CAD build for the part. Positions are in the model's coordinates, mm. Round coordinates to 2 decimals unless told otherwise and drop trailing zeros. Loops run counter-clockwise (first coordinate to the right, second up) from the corner with the lowest first, then second, coordinate; pieces in that order, holes last.
Autodesk Fusion 360 part; units mm, degrees
sketch "Sketch1" plane through (0, 0, 0) normal (0, 0, 1) x (1, 0, 0)
  line L0 (0, 0) -> (10, 0)
  line L1 (10, 0) -> (10, 10)
  line L2 (10, 10) -> (0, 10)
  line L3 (0, 10) -> (0, 0)
extrude "Extrude1" add sketch "Sketch1" along normal blind 10
fillet "Fillet1" radius 10 1 edges at (0, 5, 10)
Item 1: Cut at B-B, the plane x = 5.75. Give the cut face in (y, z).
Answers follow:
outline: (0, 0) - (10, 0) - (10, 9.05) - (0, 9.05) - close
Item 2: Probe line 1 (X direction, y = 6.5, z = 5.5); line 2 (Z direction, x = 9, y = 4.75); line 3 (Z direction, x = 2.75, y = 2). List the from-to ranges inside material, lowest first.
Answers follow:
line 1: x = 1.65 to 10
line 2: z = 0 to 9.95
line 3: z = 0 to 6.89
Item 3: Flat gauge pins, fed straight in: P1, Ø5, axis at y = 8.5, z = 9, coming from the -X side; P2, Ø3, axis at y = 2.5, z = 4.5, coming from the -X side. Where does each tip first touch, or does it go through?
Answers follow:
P1: stops at x = 2.4
P2: stops at x = 0.46
Item 4: Cut at C-C, the plane z = 7.5. Give the cut face in (x, y).
Answers follow:
outline: (3.38, 0) - (10, 0) - (10, 10) - (3.38, 10) - close
